The listing builds one solid part. Answer for the finished solid, in the listing's coordinates (mm). Coordinates: 2 decimals unless noted, no trailing zeros. Order: outer loops, then holes, each group sorted by start corner. A loop starts at its lowest first (then second) coordinate and runs counter-clockwise, first axis right, second up. Notation, with made-up numbers: (-7.75, 70) -> (33.25, 70) arc R34 cw to (33.25, 107) -> close; hole circle Ø9 at (48.25, -18). An arc over 180 degrees is marked (long way). Write item = value, one per line.
from build123d import *

# Parameters (mm, degrees)
SKETCH1_W           = 144
SKETCH1_H           = 47
BOSS_EXTRUDE1_DEPTH = 3
CUT_EXTRUDE2_DEPTH  = 10


with BuildPart() as part:
    # Sketch1 → Boss-Extrude1 (new body)
    with BuildSketch(Plane.XY):
        with Locations((87.644313661, 219.681377026)):
            Rectangle(SKETCH1_W, SKETCH1_H)
    extrude(amount=BOSS_EXTRUDE1_DEPTH)

    # Sketch5 → Cut-Extrude2 (cut)
    with BuildSketch(Plane.XY.offset(3)):
        with BuildLine():
            ThreePointArc((56.652582595, 219.681377026), (51.652582595, 224.681377026), (46.652582595, 219.681377026))
            Line((46.652582595, 219.681377026), (56.652582595, 219.681377026))
        make_face()
        with BuildLine():
            Line((56.652582595, 219.681377026), (46.652582595, 219.681377026))
            ThreePointArc((46.652582595, 219.681377026), (51.652582595, 214.681377026), (56.652582595, 219.681377026))
        make_face()
        with BuildLine():
            ThreePointArc((128.597865768, 219.681377026), (123.597865768, 224.681377026), (118.597865768, 219.681377026))
            Line((118.597865768, 219.681377026), (128.597865768, 219.681377026))
        make_face()
        with BuildLine():
            Line((128.597865768, 219.681377026), (118.597865768, 219.681377026))
            ThreePointArc((118.597865768, 219.681377026), (123.597865768, 214.681377026), (128.597865768, 219.681377026))
        make_face()
    extrude(amount=-CUT_EXTRUDE2_DEPTH, mode=Mode.SUBTRACT)


solid = part.part
Q1. Find the intervals of material crossed by line 1 along X through (y, z) = (221.5, 1.95); line 2 along Y through (x, z) = (53.5, 0.4); line 3 along X through (y, z) = (217, 0.55), in increasing order.
The answers:
line_1 = 15.64 to 47, 56.31 to 118.94, 128.26 to 159.64
line_2 = 196.18 to 215.04, 224.33 to 243.18
line_3 = 15.64 to 47.43, 55.87 to 119.38, 127.82 to 159.64
Q2. Section C-C, the plane z = 1.05 is taken. Give the vertices of the cut face in (x, y).
The answers:
outline = (15.64, 196.18) -> (159.64, 196.18) -> (159.64, 243.18) -> (15.64, 243.18) -> close; hole circle Ø10 at (51.65, 219.68); hole circle Ø10 at (123.6, 219.68)
Q3. The mould has two halves that part along X. Classify faces 1 (the face through (15.644, 219, 1)), 2 (the face through (52.303, 214.724, 1.521)), 3 (the face through (87, 243.181, 1)): released by +X, released by -X, zero draft, split by the parting line, or undercut.
The answers:
face_1 = released by -X
face_2 = undercut
face_3 = zero draft
Q4. Section B-B, the plane y = 222 is taken. Give the vertices of the cut face in (x, z), plus the area to 3 significant figures.
The answers:
outline = (15.64, 0) -> (47.22, 0) -> (47.22, 3) -> (15.64, 3) -> close; (56.08, 0) -> (119.17, 0) -> (119.17, 3) -> (56.08, 3) -> close; (128.03, 0) -> (159.64, 0) -> (159.64, 3) -> (128.03, 3) -> close
area = 379 mm2
Q5. Section A-A, the plane x = 54 is taken. Give the vertices of the cut face in (y, z), plus the area to 3 significant figures.
The answers:
outline = (196.18, 0) -> (215.27, 0) -> (215.27, 3) -> (196.18, 3) -> close; (224.1, 0) -> (243.18, 0) -> (243.18, 3) -> (224.1, 3) -> close
area = 115 mm2
